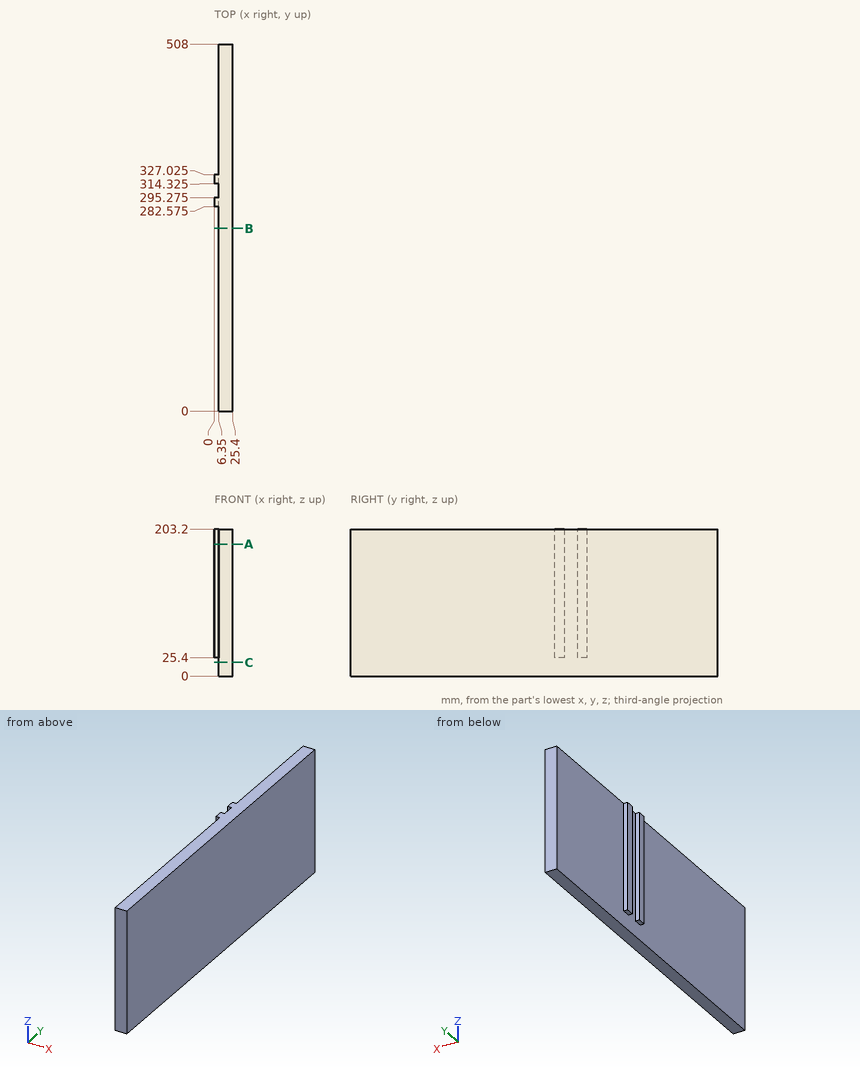
Geometry check sheet. Reference: drawing and pictorial views, mm from the part's lowest x, y, z. Give positions to 0.01 mm unless a question says otherwise; leave off trailing zeros. Order: outer loops, then holes, each group sorted by start corner. A loop starts at its lowest first (then second) coordinate and runs counter-clockwise, first axis right, second up.
1. Section check C-C, the plane z = 19. Enter the section's corners in (x, y), and give its area (3 significant figures).
2. Thickness scan on L1, parallel to Y at x = 5.5, z = 175 (3 decimals); L2, parallel to X at y = 257, z = 169.5. Record the ranges inside material, lowest first.
3. Gauge pin test, flat ends, axial feed: pin 1 Ø12 at (x, z) = (5.5, 97) entering from -Y; pin 2 Ø10 at (y, z) = (434.5, 111) entering from -X; pin 3 Ø5 at (x, z) = (2, 132) entering from -Y (3 decimals); pin 4 Ø7 at (x, z) = (2.5, 118) entering from +Y (3 decimals). Record the tip position at first contact, or that the pin passes through.
4. Section check A-A, the plane z = 182.5. Enter the section's corners in (x, y) (3 decimals), and give its area (3 significant figures).
5. Section check B-B, the plane y = 253. Enter the section's corners in (x, z), and give its area (3 significant figures).
Values follow:
1. outline: (6.35, 0) - (25.4, 0) - (25.4, 508) - (6.35, 508) - close
1. area: 9,680 mm2
2. L1: y = 282.575 to 295.275, 314.325 to 327.025
2. L2: x = 6.35 to 25.4
3. pin 1: stops at y = 0
3. pin 2: stops at x = 6.35
3. pin 3: stops at y = 282.575
3. pin 4: stops at y = 327.025
4. outline: (0, 282.575) - (6.35, 282.575) - (6.35, 0) - (25.4, 0) - (25.4, 508) - (6.35, 508) - (6.35, 327.025) - (0, 327.025) - (0, 314.325) - (6.35, 314.325) - (6.35, 295.275) - (0, 295.275) - close
4. area: 9,840 mm2
5. outline: (6.35, 0) - (25.4, 0) - (25.4, 203.2) - (6.35, 203.2) - close
5. area: 3,870 mm2
